Can you work these out from the model? Positions are in its coordinate system, mm. A direction names the side the tool comes from. Coordinates: 2 decimals unless noted, no trailing zeros. Answer as CSV lines item,"result". Start each with the question number.
1. On a 3-axis mill with a long thin cutter (end or side, diameter ignored), from which of +Z, -Z, +X, -X, +Y, -Y can I reach the whole of each face in a straight line? I mean faces 1 (the face through (-37, -13, -4)), 2 (the face through (9, 27, -8)). Say none if no direction works.
2. Will these pins go through, and if not, where does the flat tip stop? pin 1 (1.5 mm diameter, centred on x = 12, z = -3, fed in from +Y); pin 2 (1 mm diameter, centred on y = -11, z = -4.5, fed in from +X).
3. I need wall thicknesses on line 1 along Y through (x, z) = (0, -5.3); line 2 along Y through (x, z) = (-18, -4.75); line 3 along Y through (x, z) = (0, -6.6). Which ranges of each line are inside material? Lowest first, please. Write a range as from..to.
```python
from build123d import *

# Parameters (mm, degrees)
FASE1_SIZE    = 0.8
FASE2_SIZE    = 3
VERRUNDUNG1_R = 5


with BuildPart() as part:
    # Skizze3 → Rotation1 (revolve)
    with BuildSketch(Plane(origin=(0, 0, 0), x_dir=(0, 0, -1), z_dir=(1, 0, 0)), mode=Mode.PRIVATE) as rotation1_sk:
        Polygon((0, 27.5), (0, 34.9), (6, 34.9), (6, 38.1), (4, 38.1), (4, 42.5), (8, 42.5), (8, 27.5), align=None)
    revolve(rotation1_sk.sketch.rotate(Axis((0, 0, 28.082191781), (0, 0, -1)), 90), axis=Axis((0, 0, 28.082191781), (0, 0, -1)))

    # Fase1
    fase1_edges = [part.edges().sort_by_distance(p)[0] for p in [
        (-27.5, 0, -8),
        (-42.5, 0, -8),
        (-42.5, 0, -4),
        (-38.1, 0, -4),
    ]]
    chamfer(fase1_edges, length=FASE1_SIZE)

    # Fase2
    fase2_edges = [part.edges().sort_by_distance(p)[0] for p in [
        (-27.5, 0, 0),
        (-34.9, 0, 0),
    ]]
    chamfer(fase2_edges, length=FASE2_SIZE)

    # Verrundung1
    verrundung1_edges = [part.edges().sort_by_distance(p)[0] for p in [
        (-34.9, 0, -3),
        (-27.5, 0, -3),
    ]]
    fillet(verrundung1_edges, radius=VERRUNDUNG1_R)


solid = part.part
```
Solved:
1,face 1,"+Z"
1,face 2,"-Z, +X, -X, +Y, -Y"
2,pin 1,"y = 32.7"
2,pin 2,"x = 41.16"
3,line 1,"-42.5..-38.1, -34.9..-27.5, 27.5..34.9, 38.1..42.5"
3,line 2,"-38.44..-33.64, -29.89..-20.8, 20.8..29.89, 33.64..38.44"
3,line 3,"-42.5..-27.5, 27.5..42.5"
